Verification items for the finished model (mm, model axes). A direction names the side the tool comes from. Give positions to 0.01 mm unless a question says otherwise; leave off trailing zeros. Write each loop counter-clockwise with the first axis right and the second up, starting at its lowest first coordinate (ties: lowest second). Pieces come first, ordered by that corner, then holes. Notation, with made-up numbers: M 78.5,-37.75 L 108.5,-37.75 A18 cw 108.5,-21.75 Z; hole C 89,62 d8. An arc over 180 degrees is marked long. Answer as a JSON object with one key per item and string values.
```python
from build123d import *

# Parameters (mm, degrees)
SK_BOARD_W              = 56
SK_BOARD_H              = 85
EX_BOARD_DEPTH          = 1.6
SK_MOUNTHOLES_4X_R      = 1.35
CUT_MOUNTHOLES_4X_DEPTH = 1.6
SK_PORTS_USB_ETH_W      = 52
SK_PORTS_USB_ETH_H      = 24
EX_PORTS_USB_ETH_DEPTH  = 16
SK_ACTIVECOOLER_W       = 39
SK_ACTIVECOOLER_H       = 48
EX_ACTIVECOOLER_DEPTH   = 9
SK_GPIO_W               = 5
SK_GPIO_H               = 51
EX_GPIO_DEPTH           = 8.5


with BuildPart() as part:
    # SK_Board → EX_Board (new body)
    with BuildSketch(Plane(origin=(0, 0, 0), x_dir=(1, 0, 0), z_dir=(0, 1, 0))):
        Rectangle(SK_BOARD_W, SK_BOARD_H)
    extrude(amount=EX_BOARD_DEPTH)

    # SK_MountHoles_4x → CUT_MountHoles_4x (cut)
    with BuildSketch(Plane(origin=(0, 0, 0), x_dir=(1, 0, 0), z_dir=(0, 1, 0))):
        with Locations(Location((-24.5, 39, 0), (0, 0, 270))):
            Circle(SK_MOUNTHOLES_4X_R)
        with Locations(Location((24.5, 39, 0), (0, 0, 270))):
            Circle(SK_MOUNTHOLES_4X_R)
        with Locations(Location((-24.5, -19, 0), (0, 0, 270))):
            Circle(SK_MOUNTHOLES_4X_R)
        with Locations(Location((24.5, -19, 0), (0, 0, 270))):
            Circle(SK_MOUNTHOLES_4X_R)
    extrude(amount=CUT_MOUNTHOLES_4X_DEPTH, mode=Mode.SUBTRACT)

    # SK_Ports_USB_ETH → EX_Ports_USB_ETH (add)
    with BuildSketch(Plane(origin=(0, 1.6, 0), x_dir=(1, 0, 0), z_dir=(0, 1, 0))):
        with Locations((0, -33.5)):
            Rectangle(SK_PORTS_USB_ETH_W, SK_PORTS_USB_ETH_H)
    extrude(amount=EX_PORTS_USB_ETH_DEPTH)

    # SK_ActiveCooler → EX_ActiveCooler (add)
    with BuildSketch(Plane(origin=(0, 1.6, 0), x_dir=(1, 0, 0), z_dir=(0, 1, 0))):
        with Locations((-2.5, 10)):
            Rectangle(SK_ACTIVECOOLER_W, SK_ACTIVECOOLER_H)
    extrude(amount=EX_ACTIVECOOLER_DEPTH)

    # SK_GPIO → EX_GPIO (add)
    with BuildSketch(Plane(origin=(0, 1.6, 0), x_dir=(1, 0, 0), z_dir=(0, 1, 0))):
        with Locations((24.5, 10)):
            Rectangle(SK_GPIO_W, SK_GPIO_H)
    extrude(amount=EX_GPIO_DEPTH)


solid = part.part
```
1) Go/stop test with flat-tipped pins: pin 1 (3 mm diameter, centred on y = 7, z = -15, fed in from +X); pin 2 (1.5 mm diameter, centred on y = 9, z = 20.5, fed in from -X); pin 3 (4.5 mm diameter, centred on x = 24.5, z = -39, fed in from +Y); pin 4 (2.5 mm diameter, centred on x = 24.5, z = -12.5, fed in from +Y). Record where each tip stops, or that it passes through.
Completed:
{"pin 1": "stops at x = 27", "pin 2": "passes through", "pin 3": "stops at y = 1.6", "pin 4": "stops at y = 10.1"}
2) Section check C-C on x = 19. Record the boundary of the cut face in (y, z), and give its area (3 significant figures).
Completed:
{"outline": "M 0,-42.5 L 1.6,-42.5 L 1.6,21.5 L 17.6,21.5 L 17.6,45.5 L 1.6,45.5 L 1.6,42.5 L 0,42.5 Z", "area": "520 mm2"}
3) Release check for a two-part mould opening along X. For faces 1 (the face through (23.68, 0.79, -40.07)), 2 (the face through (-26, 9, 34)), 3 (the face through (-3, 6, -34)) record: pulls with the +X half, pulls with the -X half, needs draft (parallel to the pull), parting line crosses it, or undercut.
Completed:
{"face 1": "undercut", "face 2": "pulls with the -X half", "face 3": "needs draft"}
4) Section check A-A on z = 19. Record the boundary of the cut face in (x, y).
Completed:
{"outline": "M -28,0 L -25.85,0 L -25.85,1.6 L -28,1.6 Z; M -23.15,0 L 23.15,0 L 23.15,1.6 L -23.15,1.6 Z; M 25.85,0 L 28,0 L 28,1.6 L 25.85,1.6 Z"}
5) Thickness scan on L1, parallel to X at y = 0.4, z = -39; L2, parallel to X at y = 9.5, z = -26; L3, parallel to X at y = 15.25, z = 25.5. Record the ranges inside material, lowest first.
Completed:
{"L1": "x = -28 to -25.85, -23.15 to 23.15, 25.85 to 28", "L2": "x = -22 to 17, 22 to 27", "L3": "x = -26 to 26"}
6) Section check D-D on z = 9.5. Record the boundary of the cut face in (x, y), and give its area (3 significant figures).
Completed:
{"outline": "M -28,0 L 28,0 L 28,1.6 L 27,1.6 L 27,10.1 L 22,10.1 L 22,1.6 L 17,1.6 L 17,10.6 L -22,10.6 L -22,1.6 L -28,1.6 Z", "area": "483 mm2"}
7) Section check B-B on y = 6.5. Record the boundary of the cut face in (x, z), and give its area (4 significant figures).
Completed:
{"outline": "M -26,21.5 L 26,21.5 L 26,45.5 L -26,45.5 Z; M -22,-34 L 17,-34 L 17,14 L -22,14 Z; M 22,-35.5 L 27,-35.5 L 27,15.5 L 22,15.5 Z", "area": "3,375 mm2"}
8) Access from +Z, -Z, +X, -X, +Y, -Y to the whole of each face (thin tool, end or side, straight path). Record for faces 4 (the face through (27, 6, -10)), 5 (the face through (17, 6, -10)), 6 (the face through (24, 10.1, -10)), 7 (the face through (24, 6, 15.5)), 8 (the face through (0, 1.6, 44)).
Completed:
{"face 4": "+Z, -Z, +X, +Y", "face 5": "-Z, +Y", "face 6": "-Z, +X, +Y", "face 7": "+X, -X, +Y", "face 8": "+Z, +X, -X, -Y"}
